CAD build for the part. Positions are in the model's coordinates, mm. A direction names the side the tool comes from. Round coordinates to 2 decimals unless told otherwise and drop trailing zeros. Order: outer loops, then holes, each group sorted by start corner. A loop starts at its lowest first (then second) coordinate and runs counter-clockwise, first axis right, second up. Notation, with made-up numbers: M 46,-31 L 87,-31 A27 ccw 87,-8 Z; hole C 86,-1 d5. An arc over 180 degrees is marked long. Answer as a JSON object with one key per item and string values.
```python
from build123d import *

# Parameters (mm, degrees)
F3_DEPTH = 15
F4_DEPTH = 15
F5_DEPTH = 15
F7_R     = 1


# Not quite as in the source:
# - after a boolean that leaves OpenCascade's solid faulty, fix() repairs it
# - a feature of the source that left no trace in its solid (it failed there, or was rolled back) is left out


with BuildPart() as f1:
    # F0 (on Front) → F1 (revolve)
    with BuildSketch(Plane.XZ):
        Polygon((2.7639019594, 2.7772041211), (2.7639019594, 1.666), (15.7639019594, 1.666), (15.7639019594, 2.3962433916), (15.2639019594, 2.9), (11.4639019594, 2.9), (10.9639019594, 3.1), (10.4639019594, 2.9), (5.7639019594, 2.9), (5.7639019594, 5), (3.7639019594, 5), (3.7639019594, 2.7772041211), align=None)
    revolve(axis=Axis((8.0730360566, 0, 0), (1, 0, 0)))

    # F2 (on face) → F3 (join)
    with BuildSketch(Plane(origin=(2.7639019594, 0, 0), x_dir=(0, -1, 0), z_dir=(-1, 0, 0))):
        with BuildLine():
            ThreePointArc((-1.1878670343, 1.1681300907), (-0.7352206258, 1.4949938566), (-0.2, 1.6539516317))
            Line((-0.2, 1.6539516317), (-0.2, 2.7699932726))
            ThreePointArc((-0.2, 2.7699932726), (-1.249471885, 2.4802586032), (-2.1069209339, 1.8093498579))
            ThreePointArc((-2.1069209339, 1.8093498579), (-2.5677957056, 1.0579640563), (-2.7699932726, 0.2))
            Line((-2.7699932726, 0.2), (-1.6539516317, 0.2))
            ThreePointArc((-1.6539516317, 0.2), (-1.5011003633, 0.7226712249), (-1.1878670343, 1.1681300907))
        make_face()
    extrude(amount=F3_DEPTH)

    # F2 (on face) → F4 (join)
    with BuildSketch(Plane(origin=(2.7639019594, 0, 0), x_dir=(0, -1, 0), z_dir=(-1, 0, 0))):
        with BuildLine():
            Line((0.2, 2.7699932726), (0.2, 1.6539516317))
            ThreePointArc((0.2, 1.6539516317), (0.75564146, 1.4847767455), (1.2194377654, 1.1351332681))
            ThreePointArc((1.2194377654, 1.1351332681), (1.5108640621, 0.7020297614), (1.6539516317, 0.2))
            Line((1.6539516317, 0.2), (2.7699932726, 0.2))
            ThreePointArc((2.7699932726, 0.2), (2.5121240066, 1.1841012226), (1.917164961, 2.0093136247))
            ThreePointArc((1.917164961, 2.0093136247), (1.1248356545, 2.5392139493), (0.2, 2.7699932726))
        make_face()
    extrude(amount=F4_DEPTH)

    # F2 (on face) → F5 (join)
    with BuildSketch(Plane(origin=(2.7639019594, 0, 0), x_dir=(0, -1, 0), z_dir=(-1, 0, 0))):
        with BuildLine():
            ThreePointArc((-1.1878670343, 1.1681300907), (-0.7352206258, 1.4949938566), (-0.2, 1.6539516317))
            Line((-0.2, 1.6539516317), (-0.2, 2.7699932726))
            ThreePointArc((-0.2, 2.7699932726), (-1.249471885, 2.4802586032), (-2.1069209339, 1.8093498579))
            ThreePointArc((-2.1069209339, 1.8093498579), (-2.5677957056, 1.0579640563), (-2.7699932726, 0.2))
            Line((-2.7699932726, 0.2), (-1.6539516317, 0.2))
            ThreePointArc((-1.6539516317, 0.2), (-1.5011003633, 0.7226712249), (-1.1878670343, 1.1681300907))
        make_face()
        with BuildLine():
            Line((0.2, 2.7699932726), (0.2, 1.6539516317))
            ThreePointArc((0.2, 1.6539516317), (0.75564146, 1.4847767455), (1.2194377654, 1.1351332681))
            ThreePointArc((1.2194377654, 1.1351332681), (1.5108640621, 0.7020297614), (1.6539516317, 0.2))
            Line((1.6539516317, 0.2), (2.7699932726, 0.2))
            ThreePointArc((2.7699932726, 0.2), (2.5121240066, 1.1841012226), (1.917164961, 2.0093136247))
            ThreePointArc((1.917164961, 2.0093136247), (1.1248356545, 2.5392139493), (0.2, 2.7699932726))
        make_face()
        with BuildLine():
            ThreePointArc((-0.2, -1.6539516317), (-1.1780398975, -1.1780398975), (-1.6539516317, -0.2))
            Line((-1.6539516317, -0.2), (-2.7699932726, -0.2))
            ThreePointArc((-2.7699932726, -0.2), (-1.9637798667, -1.9637798667), (-0.2, -2.7699932726))
            Line((-0.2, -2.7699932726), (-0.2, -1.6539516317))
        make_face()
        with BuildLine():
            Line((2.7699932726, -0.2), (1.6539516317, -0.2))
            ThreePointArc((1.6539516317, -0.2), (1.1780398975, -1.1780398975), (0.2, -1.6539516317))
            Line((0.2, -1.6539516317), (0.2, -2.7699932726))
            ThreePointArc((0.2, -2.7699932726), (1.9637798667, -1.9637798667), (2.7699932726, -0.2))
        make_face()
    extrude(amount=F5_DEPTH)

    add(f1.part.fix(), mode=Mode.REPLACE)

    # F7
    f7_edges = [f1.edges().sort_by_distance(p)[0] for p in [
        (3.763902, 0, -5),
    ]]
    fillet(f7_edges, radius=F7_R)


solid = f1.part
```
Item 1: Saw through at A-A on x = -8.5. List the corners of the cut face in (y, z).
Worked answers:
{"outline": "M -2.77,-0.2 A2.78 ccw -0.2,-2.77 L -0.2,-1.65 A1.67 cw -1.65,-0.2 Z; M -2.77,0.2 L -1.65,0.2 A1.67 cw -0.2,1.65 L -0.2,2.77 A2.78 ccw Z; M 0.2,-2.77 A2.78 ccw 2.77,-0.2 L 1.65,-0.2 A1.67 cw 0.2,-1.65 Z; M 0.2,1.65 A1.67 cw 1.65,0.2 L 2.77,0.2 A2.78 ccw 0.2,2.77 Z"}
Item 2: Drop flat-ended pins along their axis: pin 1 Ø0.6 at (x, z) = (-6, 2.5) entering from +Y; pin 2 Ø6 at (x, y) = (12.5, 2.5) entering from -Z; pin 3 Ø0.6 at (x, z) = (-6, 2) entering from -Y; pin 4 Ø1 at (x, y) = (-7, 3.5) entering from -Z. Give the stop position or say it passes through.
Worked answers:
{"pin 1": "stops at y = 1.69", "pin 2": "stops at z = -3.1", "pin 3": "stops at y = -2.2", "pin 4": "passes through"}
Item 3: Wall check: line 1 along Z through (x, y) = (7.75, 0); line 2 along Y through (x, z) = (10.75, 0). Give the ranges that are in metal, low to high. Write a range as [from, to].
Worked answers:
{"line 1": "z = [-2.9, -1.67], [1.67, 2.9]", "line 2": "y = [-3.01, -1.67], [1.67, 3.01]"}
Item 4: Two-plate mould, pull along Z, no slides. Class faces 1 (the flat face through (-12.236, 1.5, 1.5)), 2 (the flat face through (-5, -2, -0.2)), 3 (the cylindrical face through (8.1, -0.1, -2.9)): released by +Z, released by -Z, zero draft, split by the parting line, or undercut.
Worked answers:
{"face 1": "zero draft", "face 2": "undercut", "face 3": "split by the parting line"}
Item 5: 3-axis set-ups, long thin cutter, end or side, ignore diameter. For faces 4 (the cylindrical face through (13.3, -0.1, -2.9)), 5 (the flat face through (-5, -2, 0.2)), 6 (the flat face through (15.764, -2, 0)), 7 (the flat face through (-5, 0.2, -2)), 8 (the flat face through (3.764, -3, 1)): which of +Z, -Z, +X, -X, +Y, -Y reach the whole face in a straight line?
Worked answers:
{"face 4": "+X", "face 5": "-X, +Y, -Y", "face 6": "+Z, -Z, +X, +Y, -Y", "face 7": "+Z, -Z, -X", "face 8": "-X"}
